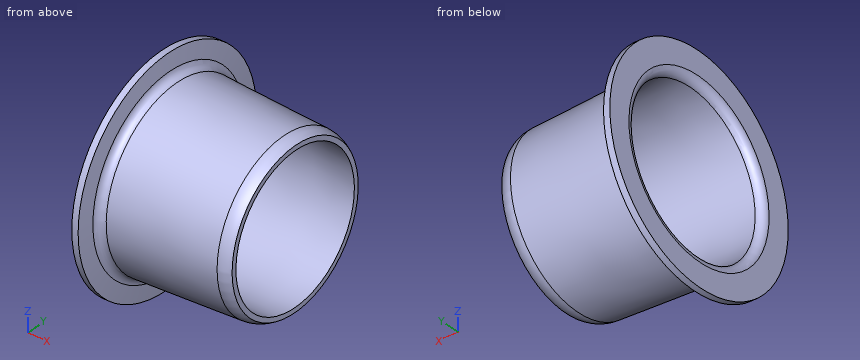
```python
from build123d import *


with BuildPart() as part:
    # Esboço1 → Revolução1 (revolve)
    with BuildSketch(Plane.XY, mode=Mode.PRIVATE) as revolu_o1_sk:
        with BuildLine():
            Line((0, 2.199809904), (0, 2.8))
            Line((0, 2.8), (0.16, 2.8))
            Line((0.16, 2.8), (0.196537584, 2.382373504))
            ThreePointArc((0.196537584, 2.382373504), (0.257432856, 2.255371175), (0.386939067, 2.2))
            Line((0.386939067, 2.2), (3.1, 2.08))
            ThreePointArc((3.1, 2.08), (3.256983611, 2.050950832), (3.4, 1.98))
            Line((3.4, 1.98), (3.4, 1.86))
            Line((3.4, 1.86), (0.191282067, 2))
            ThreePointArc((0.191282067, 2), (0.055529265, 2.061505143), (0, 2.199809904))
        make_face()
    revolve(revolu_o1_sk.sketch.rotate(Axis((0, 0, 0), (1, 0, 0)), 90), axis=Axis((0, 0, 0), (1, 0, 0)))


solid = part.part
```
Geometry check sheet. Reference: the model listing, model coordinates, mm. Coordinates: 2 decimals unless noted, no trailing zeros. Write each loop counter-clockwise with the first axis right and the second up, starting at its lowest first coordinate (ties: lowest second). Pieces come first, ordered by that corner, then holes. Notation, with made-up numbers: M -1,-11 L 10,-11 A19 ccw 10,-4 Z; hole C 16,-2 d1. An arc over 180 degrees is marked long. One line per item, written item: value. Start each with the question number.
(1) Depth check by flat-ended pin: pin 1 (1 mm diameter, centred on x = 3, y = -1, fed in from -Z); pin 2 (2 mm diameter, centred on x = 3, y = -2, fed in from +Z). Enter the tip coordinate at first touch or a pass-through.
(2) Sectioned sample at A-A, the plane z = 0. Enter the section's corners in (x, y), and give its area (3 significant figures).
(3) Sectioned sample at D-D, the plane x = 0.5. Enter the section's corners in (y, z) (3 decimals), and give its area (3 significant figures).
(4) Scan lines: line 1 along Y through (x, z) = (1.7, -0.1); line 2 along Z through (x, y) = (2.55, -0.9); line 3 along Y through (x, z) = (1.35, 1.25). Record each from-to range of solid material in increasing order. Write a range as [from, to].
(5) Sectioned sample at C-C, the plane x = 2.6. Enter the section's corners in (y, z), and give its area (3 significant figures).
Filled sheet:
1. pin 1: z = -2.03
1. pin 2: z = 1.83
2. outline: M 0,-2.8 L 0.16,-2.8 L 0.2,-2.38 A0.2 cw 0.39,-2.2 L 3.1,-2.08 A0.58 ccw 3.4,-1.98 L 3.4,-1.86 L 0.19,-2 A0.2 ccw 0,-2.2 Z; M 0,2.2 A0.2 ccw 0.19,2 L 3.4,1.86 L 3.4,1.98 A0.58 ccw 3.1,2.08 L 0.39,2.2 A0.2 cw 0.2,2.38 L 0.16,2.8 L 0,2.8 Z
2. area: 1.61 mm²
3. outline: C 0,0 d4.39; hole C 0,0 d3.973
3. area: 2.74 mm²
4. line 1: [-2.14, -1.93], [1.93, 2.14]
4. line 2: [-1.9, -1.67], [1.67, 1.9]
4. line 3: [-1.76, -1.5], [1.5, 1.76]
5. outline: C 0,0 d4.2; hole C 0,0 d3.79
5. area: 2.60 mm²
